Can you work these out from the model? Positions are in its coordinate system, mm. A direction names the side the tool comes from. Coordinates: 2 decimals unless noted, no trailing zeros. Order: outer loops, then holes, each group sorted by start corner. A loop starts at its lowest first (then second) coordinate and runs counter-clockwise, first axis right, second up. Notation, with made-up numbers: (31, 23) -> (47, 23) arc R17 ccw to (47, 30) -> close; hole circle Ø3 at (-10.75, 16). An arc over 180 degrees is marked (long way). Answer in a Markdown table with one row per item.
```python
from build123d import *

# Parameters (mm, degrees)
EXTRUDE_THIN3_DEPTH      = 6
EXTRUDE_THIN3_DEPTH_BACK = 0.2
EXTRUDE1_REACH           = 23.681
SKETCH2_R                = 1.25


with BuildPart() as part:
    # Sketch1 → Extrude-Thin3 (new, two sides: drawn at the far end of the back side and taken through both)
    with BuildSketch(Plane(origin=(0, 0, 0), x_dir=(1, 0, 0), z_dir=(0, 1, 0)).offset(-EXTRUDE_THIN3_DEPTH_BACK)):
        with BuildLine():
            Line((-5.502320154, 18.122508758), (-3.972308472, 15.827491235))
            ThreePointArc((-3.972308472, 15.827491235), (-3.86802113, 15.387436777), (-4.076023457, 14.985866351))
            ThreePointArc((-4.076023457, 14.985866351), (-6.044162598, 10.047161593), (-3.362094774, 5.456857838))
            ThreePointArc((-3.362094774, 5.456857838), (-2.89934417, 4.166748229), (-4, 3.35))
            Line((-4, 3.35), (-7, 3.35))
            ThreePointArc((-7, 3.35), (-8.85, 1.5), (-7, -0.35))
            Line((-7, -0.35), (7, -0.35))
            ThreePointArc((7, -0.35), (8.85, 1.5), (7, 3.35))
            Line((7, 3.35), (4, 3.35))
            ThreePointArc((4, 3.35), (2.89934417, 4.166748229), (3.362094774, 5.456857838))
            ThreePointArc((3.362094774, 5.456857838), (6.044162598, 10.047161593), (4.076023457, 14.985866351))
            ThreePointArc((4.076023457, 14.985866351), (3.86802113, 15.387436777), (3.972308472, 15.827491235))
            Line((3.972308472, 15.827491235), (5.502320154, 18.122508758))
            Line((5.502320154, 18.122508758), (4.919884948, 18.510798895))
            Line((4.919884948, 18.510798895), (3.389873266, 16.215781372))
            ThreePointArc((3.389873266, 16.215781372), (3.17327648, 15.301822114), (3.605281311, 14.467791228))
            ThreePointArc((3.605281311, 14.467791228), (5.346119002, 10.099460144), (2.973804637, 6.039293045))
            ThreePointArc((2.973804637, 6.039293045), (2.229379751, 3.963899325), (4, 2.65))
            Line((4, 2.65), (7, 2.65))
            ThreePointArc((7, 2.65), (8.15, 1.5), (7, 0.35))
            Line((7, 0.35), (-7, 0.35))
            ThreePointArc((-7, 0.35), (-8.15, 1.5), (-7, 2.65))
            Line((-7, 2.65), (-4, 2.65))
            ThreePointArc((-4, 2.65), (-2.229379751, 3.963899325), (-2.973804637, 6.039293045))
            ThreePointArc((-2.973804637, 6.039293045), (-5.346119002, 10.099460144), (-3.605281311, 14.467791228))
            ThreePointArc((-3.605281311, 14.467791228), (-3.17327648, 15.301822114), (-3.389873266, 16.215781372))
            Line((-3.389873266, 16.215781372), (-4.919884948, 18.510798895))
            Line((-4.919884948, 18.510798895), (-5.502320154, 18.122508758))
        make_face()
    extrude(amount=EXTRUDE_THIN3_DEPTH + EXTRUDE_THIN3_DEPTH_BACK)

    # Sketch2 → Extrude1 (cut, up to next)
    with BuildSketch(Plane.XY.offset(0.35), mode=Mode.PRIVATE) as extrude1_sk1:
        with Locations((0, 3)):
            Circle(SKETCH2_R)
    extrude1_tool1 = extrude(extrude1_sk1.sketch, amount=-EXTRUDE1_REACH, mode=Mode.PRIVATE) & part.part
    add(extrude1_tool1.solids().sort_by_distance((0, 3, 0.35))[0], mode=Mode.SUBTRACT)


solid = part.part
```
(1) On a 3-axis mill with a long thin cutter (end or side, diameter ignored), from which of +Z, -Z, +X, -X, +Y, -Y can I reach the whole of each face in a straight line? I mean faces 1 (the flat face through (2.6, -0.2, -4.9)), 2 (the flat face through (6, 3, -3.35)), 3 (the cylindrical face through (-5.34, 2.86, -10.03)), 4 (the flat face through (-4.748, 2.857, -16.991)). Say none if no direction works.
Response values:
| item | result |
|---|---|
| face 1 | +Z, -Z, +X, -X, -Y |
| face 2 | +X, +Y, -Y |
| face 3 | +Y, -Y |
| face 4 | -X, +Y, -Y |
(2) We'd pull the mould along Z, two halves only. Please class faces 5 (the cylindrical face through (8.85, 2.86, -1.46)), 6 (the flat face through (-4.144, 2.857, -17.347)), 7 (the cylindrical face through (-0.16, 4.24, 0)), 8 (the cylindrical face through (8.15, 2.86, -1.53)): +Z half, -Z half, draft (parallel to the pull), parting line (faces both ways), or undercut.
Response values:
| item | result |
|---|---|
| face 5 | parting line |
| face 6 | -Z half |
| face 7 | draft |
| face 8 | undercut |
(3) Suppose I cut it at D-D (y = 1.5). Please give me the cut outline in (x, z).
Response values:
| item | result |
|---|---|
| outline | (-7, -3.35) -> (-4, -3.35) arc R1.15 cw to (-3.36, -5.46) arc R6.06 ccw to (-4.08, -14.99) arc R0.65 cw to (-3.97, -15.83) -> (-5.5, -18.12) -> (-4.92, -18.51) -> (-3.39, -16.22) arc R1.35 ccw to (-3.61, -14.47) arc R5.36 cw to (-2.97, -6.04) arc R1.85 ccw to (-4, -2.65) -> (-7, -2.65) arc R1.15 cw to (-7, -0.35) -> (7, -0.35) arc R1.15 cw to (7, -2.65) -> (4, -2.65) arc R1.85 ccw to (2.97, -6.04) arc R5.36 cw to (3.61, -14.47) arc R1.35 ccw to (3.39, -16.22) -> (4.92, -18.51) -> (5.5, -18.12) -> (3.97, -15.83) arc R0.65 cw to (4.08, -14.99) arc R6.06 ccw to (3.36, -5.46) arc R1.15 cw to (4, -3.35) -> (7, -3.35) arc R1.85 ccw to (7, 0.35) -> (-7, 0.35) arc R1.85 ccw to start |
(4) I need wall thicknesses on line 1 (Y direction, x = 0, z = -0.1); line 2 (Z direction, x = -6.5, y = 0.5); line 3 (Z direction, x = 3.5, y = 0.5). Which ranges of each line are inside material? Lowest first, please. Write a range as [from, to].
Response values:
| item | result |
|---|---|
| line 1 | [-0.2, 1.75], [4.25, 6] |
| line 2 | [-3.35, -2.65], [-0.35, 0.35] |
| line 3 | [-16.38, -14.57], [-6.44, -5.55], [-3.46, -2.72], [-0.35, 0.35] |
(5) Suppose I cut it at B-B (z = -1.5). Please give me the cut outline in (x, y), and give its area (3 significant figures).
Response values:
| item | result |
|---|---|
| outline | (-8.85, -0.2) -> (-8.15, -0.2) -> (-8.15, 6) -> (-8.85, 6) -> close; (8.15, -0.2) -> (8.85, -0.2) -> (8.85, 6) -> (8.15, 6) -> close |
| area | 8.68 mm2 |
(6) Will these pins go through, and if not, where does the flat tip stop? pin 1 Ø1 at (y, z) = (4.5, -8.5) entering from +X; pin 2 Ø3 at (x, y) = (0, 3) entering from -Z; pin 3 Ø3 at (x, y) = (-1.5, 3) entering from -Z.
Response values:
| item | result |
|---|---|
| pin 1 | x = 5.87 |
| pin 2 | z = -0.35 |
| pin 3 | z = -6.06 |
(7) Suppose I cut it at A-A (x = 0). Please give me the cut outline in (y, z), and give its area (3 significant figures).
Response values:
| item | result |
|---|---|
| outline | (-0.2, -0.35) -> (1.75, -0.35) -> (1.75, 0.35) -> (-0.2, 0.35) -> close; (4.25, -0.35) -> (6, -0.35) -> (6, 0.35) -> (4.25, 0.35) -> close |
| area | 2.59 mm2 |
